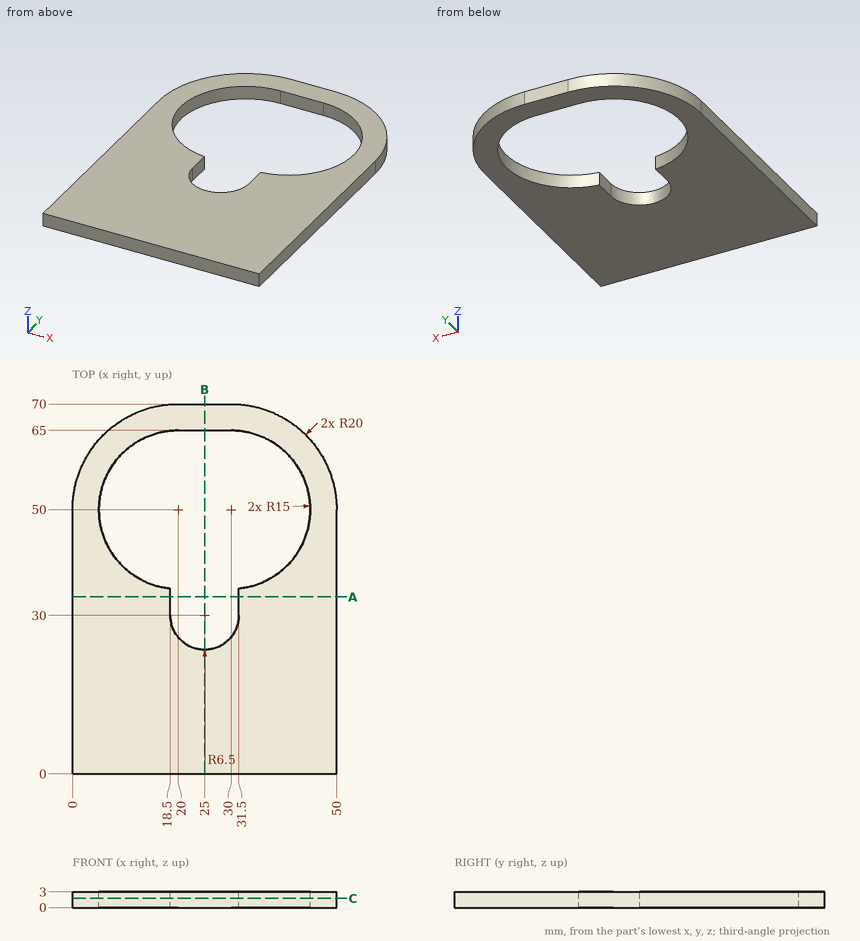
Drawing for the job (mm, zero at the part's lowest x, y, z). Round coordinates to 2 decimals unless told otherwise and drop trailing zeros. Write each loop counter-clockwise with the first axis right and the second up, starting at its lowest first coordinate (ties: lowest second). Pieces come first, ordered by that corner, then holes. Notation, with made-up numbers: M 72.25,-32.75 L 124.25,-32.75 A12 cw 124.25,-20.75 Z; hole C -3.5,80.25 d3. An arc over 180 degrees is marked long. Answer as a JSON object with one key per item and string values. Group by question number.
(1) Drill centre lines: L1, parallel to X at y = 63.5, z = 1.5; L2, parallel to Y at x = 39.5, z = 2.8; L3, parallel to Y at x = 6.5, z = 2.5. Where is each one in solid material? Low to high.
(2) Cut at B-B (x = 25). Give the cut face in (y, z).
(3) Cut at C-C (z = 1.75). Give the cut face in (x, y).
(4) Cut at A-A (y = 33.5). Give the cut face in (x, z).
(5) Flat gauge pin, fed straight in: pin 1 (1.5 mm diameter, centred on x = 41.5, z = 1, fed in from -Y). Where does the tip first touch, or does it go through?
Responses:
{
 "1": {"L1": "x = 5.24 to 13.46, 36.54 to 44.76", "L2": "y = 0 to 38.39, 61.61 to 67.6", "L3": "y = 0 to 43.46, 56.54 to 64.76"},
 "2": {"outline": "M 0,0 L 23.5,0 L 23.5,3 L 0,3 Z; M 65,0 L 70,0 L 70,3 L 65,3 Z"},
 "3": {"outline": "M 0,0 L 50,0 L 50,50 A20 ccw 30,70 L 20,70 A20 ccw 0,50 Z; hole M 18.5,30 A6.5 ccw 31.5,30 L 31.5,35.08 A15 ccw 30,65 L 20,65 A15 ccw 18.5,35.08 Z"},
 "4": {"outline": "M 0,0 L 18.5,0 L 18.5,3 L 0,3 Z; M 31.5,0 L 50,0 L 50,3 L 31.5,3 Z"},
 "5": {"pin 1": "stops at y = 0"}
}
